Read the model definition and answer for the solid it produces. Units are mm, in the model's axes. Coordinates: 2 decimals unless noted, no trailing zeros. Order: outer loops, then holes, each group sorted by start corner. A loop starts at its lowest first (then second) coordinate and runs counter-clockwise, first axis right, second up. Notation, with made-up numbers: M -38,86.5 L 10,86.5 A31 ccw 10,123.5 Z; hole C 38.25,60.5 d8. An arc over 180 degrees is marked long. Use a Markdown table: item, result. Add a question column.
1) Find the intervals of material crossed by probe 1 along Y at (x, z) = (-72.25, 4.25); probe 2 along X at (y, z) = (46.25, 2.5); probe 3 along Z at (x, y) = (-75.75, 40.25), in increasing order. Write a range as [from, to].
2) The mould has two halves that part along Y. Classify faces 1 (the face through (-72.73, 45.65, 3.72)), 2 (the face through (-69, 42, 0)), 3 (the face through (-74.659, 40.354, 0.493)), 4 (the face through (-73.255, 49.616, 3.211)): released by +Y, released by -Y, zero draft, split by the parting line, or undercut.
3) Find section A-A on z = 6.25. Write down the section's boundary in (x, y), plus the area to 3 significant figures.
4) Find section B-B on z = 2.25. Write down the section's boundary in (x, y).
5) Each of these flat-tipped pins is pushed along its axis until it touches: pin 1 Ø3 at (y, z) = (45.5, 3) entering from +X; pin 2 Ø8 at (x, y) = (-66.5, 39) entering from -Z; pin 3 Ø5 at (x, y) = (-72.28, 42.18) entering from +Z; pin 4 Ø2 at (x, z) = (-77, 1) entering from -Y. Where does it stop, or does it pass through?
from build123d import *

# Parameters (mm, degrees)
F0_R     = 7.5
F0_R_2   = 3.5
F1_DEPTH = 6.5
F0_R_3   = 3
F2_DEPTH = 1.5
F3_SIZE  = 0.49999


# Not quite as in the source:
# - a fillet or chamfer is up to 0.001 mm smaller than in the source, because OpenCascade refuses the exact size


with BuildPart() as f1:
    # F0 (on Top) → F1 (new body)
    with BuildSketch(Plane.XY):
        with Locations((-72.2782313824, 42.1795584261)):
            Circle(F0_R)
        with Locations((-72.2782313824, 42.1795584261)):
            Circle(F0_R_2, mode=Mode.SUBTRACT)
    extrude(amount=F1_DEPTH)

    # F0 (on Top) → F2 (join)
    with BuildSketch(Plane.XY):
        with Locations((-72.2782313824, 42.1795584261)):
            Circle(F0_R_2)
        with Locations((-72.2782313824, 42.1795584261)):
            Circle(F0_R_3, mode=Mode.SUBTRACT)
    extrude(amount=F2_DEPTH)

    # F3 (size 0.5 in the source; OpenCascade refuses exactly that, so slightly less here)
    f3_edges = [f1.edges().sort_by_distance(p)[0] for p in [
        (-79.778231, 42.179558, 6.5),
        (-75.778231, 42.179558, 6.5),
        (-75.278231, 42.179558, 1.5),
        (-79.778231, 42.179558, 0),
    ]]
    chamfer(f3_edges, length=F3_SIZE)


solid = f1.part
Check result:
| question | item | result |
|---|---|---|
| 1 | probe 1 | y = [34.68, 38.68], [45.68, 49.68] |
| 1 | probe 2 | x = [-78.58, -65.98] |
| 1 | probe 3 | z = [0, 6.47] |
| 2 | face 1 | undercut |
| 2 | face 2 | zero draft |
| 2 | face 3 | undercut |
| 2 | face 4 | split by the parting line |
| 3 | outline | C -72.28,42.18 d14.5; hole C -72.28,42.18 d7.5 |
| 3 | area | 121 mm2 |
| 4 | outline | C -72.28,42.18 d15; hole C -72.28,42.18 d7 |
| 5 | pin 1 | stops at x = -65 |
| 5 | pin 2 | stops at z = 0 |
| 5 | pin 3 | passes through |
| 5 | pin 4 | stops at y = 35.67 |
